from build123d import *

# Parameters (mm, degrees)
IZIM1_R                     = 10
Y_KSEKLIK_EKSTR_ZYON1_DEPTH = 25
RADYUS1_R                   = 20
RADYUS2_R                   = 100
PAH1_SIZE                   = 2
KES_EKSTR_ZYON1_DEPTH       = 276.643654753
KES_EKSTR_ZYON1_DEPTH_BACK  = 276.643654753
RADYUS3_R                   = 3


with BuildPart() as part:
    # Çizim1 → Yükseklik-Ekstrüzyon1 (new body)
    with BuildSketch(Plane.XY):
        with BuildLine():
            Line((-37.396370289, 12.396370289), (-12.396370289, 12.396370289))
            Line((-12.396370289, 12.396370289), (12.396370289, -12.396370289))
            Line((12.396370289, -12.396370289), (12.396370289, -182.396370289))
            Line((12.396370289, -182.396370289), (47.759074277, -243.646370289))
            ThreePointArc((47.759074277, -243.646370289), (41.353629711, -267.551814855), (17.448185145, -261.146370289))
            Line((17.448185145, -261.146370289), (-33.791651246, -172.396370289))
            Line((-33.791651246, -172.396370289), (-12.603629711, -154.617509234))
            Line((-12.603629711, -154.617509234), (-12.603629711, -57.396370289))
            Line((-12.603629711, -57.396370289), (-37.396370289, -32.603629711))
            Line((-37.396370289, -32.603629711), (-37.396370289, 12.396370289))
        make_face()
        with Locations((-7.396370289, -177.396370289)):
            Circle(IZIM1_R, mode=Mode.SUBTRACT)
        with Locations((32.603629711, -252.396370289)):
            Circle(IZIM1_R, mode=Mode.SUBTRACT)
    extrude(amount=Y_KSEKLIK_EKSTR_ZYON1_DEPTH)

    # Radyus1
    radyus1_edges = [part.edges().sort_by_distance(p)[0] for p in [
        (-33.791651246, -172.396370289, 12.5),
        (-12.603629711, -154.617509234, 12.5),
        (-12.603629711, -57.396370289, 12.5),
    ]]
    fillet(radyus1_edges, radius=RADYUS1_R)

    # Radyus2
    radyus2_edges = [part.edges().sort_by_distance(p)[0] for p in [
        (12.396370289, -182.396370289, 12.5),
    ]]
    fillet(radyus2_edges, radius=RADYUS2_R)

    # Pah1
    pah1_edges = [part.edges().sort_by_distance(p)[0] for p in [
        (-17.396370289, -177.396370289, 0),
        (-17.396370289, -177.396370289, 25),
        (22.603629711, -252.396370289, 0),
        (22.603629711, -252.396370289, 25),
    ]]
    chamfer(pah1_edges, length=PAH1_SIZE)

    # Çizim2 → Kes-Ekstrüzyon1 (cut, two sides: drawn at the far end of the back side and taken through both)
    with BuildSketch(Plane(origin=(0, 0, 0), x_dir=(-1, 0, 0), z_dir=(0, 0, -1)).offset(-KES_EKSTR_ZYON1_DEPTH_BACK)):
        Polygon((37.396370289, 12.396370289), (37.396370289, 10.396370289), (35.896370289, 8.896370289), (37.396370289, 7.396370289), (37.396370289, 5.396370289), (35.896370289, 3.896370289), (37.396370289, 2.396370289), (37.396370289, 0.396370289), (35.896370289, -1.103629711), (37.396370289, -2.603629711), (37.396370289, -4.603629711), (35.896370289, -6.103629711), (37.396370289, -7.603629711), (37.396370289, -9.603629711), (35.896370289, -11.103629711), (37.396370289, -12.603629711), (37.396370289, -14.603629711), (35.896370289, -16.103629711), (37.396370289, -17.603629711), (37.396370289, -19.603629711), (35.896370289, -21.103629711), (37.396370289, -22.603629711), (37.396370289, -24.603629711), (35.896370289, -26.103629711), (37.396370289, -27.603629711), (37.396370289, -29.603629711), (35.896370289, -31.103629711), (37.396370289, -32.603629711), (40.97255524, -32.603629711), (40.97255524, 12.396370289), align=None)
    extrude(amount=KES_EKSTR_ZYON1_DEPTH + KES_EKSTR_ZYON1_DEPTH_BACK, mode=Mode.SUBTRACT)

    # Radyus3
    radyus3_edges = [part.edges().sort_by_distance(p)[0] for p in [
        (-27.928932188, -42.071067812, 25),
        (-14.126039061, -58.026972889, 25),
        (-12.603629711, -105.485998804, 25),
        (-14.47747397, -153.743721305, 25),
        (-20.341888285, -161.110679149, 25),
        (-27.776301919, -173.457038674, 25),
        (-3.976234895, -224.038186258, 25),
        (41.353629711, -267.551814855, 25),
        (36.776452094, -224.623910668, 25),
        (15.80378766, -181.483355556, 25),
        (-27.928932188, -42.071067812, 0),
        (-14.126039061, -58.026972889, 0),
        (-12.603629711, -105.485998804, 0),
        (-14.47747397, -153.743721305, 0),
        (-20.341888285, -161.110679149, 0),
        (-27.776301919, -173.457038674, 0),
        (-3.976234895, -224.038186258, 0),
        (41.353629711, -267.551814855, 0),
        (36.776452094, -224.623910668, 0),
        (15.80378766, -181.483355556, 0),
        (12.396370289, -83.998910668, 25),
        (0, 0, 25),
        (-24.896370289, 12.396370289, 25),
        (-24.896370289, 12.396370289, 0),
        (12.396370289, -83.998910668, 0),
        (0, 0, 0),
    ]]
    fillet(radyus3_edges, radius=RADYUS3_R)


solid = part.part
Verification items for the finished model (mm, model axes). A direction names the side the tool comes from. Coordinates: 2 decimals unless noted, no trailing zeros. Loops run counter-clockwise (first coordinate to the right, second up) from the corner with the lowest first, then second, coordinate; pieces in that order, holes last. Notation, with made-up numbers: M 75.5,-21 L 92.5,-21 A27 ccw 92.5,-1 Z; hole C 50,63.5 d9. An arc over 180 degrees is marked long. One line per item, written item: value.
1. Gauge pin test, flat ends, axial feed: P1, Ø3, axis at x = -19, y = -179.5, coming from the +Z side; P2, Ø10, axis at x = 19.5, z = 5.5, coming from the -Y side; P3, Ø9.5, axis at y = -117, z = 8, coming from the -X side; P4, Ø1, axis at x = 37.5, z = 20, coming from the +Y side. Record the tip position at first contact, or that the pin passes through.
Answers follow:
P1: z = 25
P2: y = -267.91
P3: x = -12.6
P4: y = -225.01
2. Mould release check, pull along Y, two halves, no side actions. Record for faces 3 (the cylindrical face through (-14.168, -57.926, 12.633)), 4 (the cylindrical face through (-28.5, -40.23, 0.86)), 5 (the flat face through (-25, 12.396, 12)), 6 (the flat face through (12.396, -83, 12)): pulls with the +Y half, pulls with the -Y half, needs draft (parallel to the pull), parting line crosses it, or undercut.
Answers follow:
face 3: undercut
face 4: undercut
face 5: pulls with the +Y half
face 6: needs draft
3. Section check B-B on z = 7.75. Give the number of separate pieces and of enclosed holes in the cut face, plus the area to 3 significant figures.
Answers follow:
separate pieces: 1
enclosed holes: 2
area: 9,040 mm^2
4. Section check A-A on y = -92. Record the cut outline in (x, z).
Answers follow:
outline: M -12.6,3 A3 ccw -9.6,0 L 9.4,0 A3 ccw 12.4,3 L 12.4,22 A3 ccw 9.4,25 L -9.6,25 A3 ccw -12.6,22 Z
5. Set-up check for faces 1 (the conical face through (-1.953, -168.859, 23.125)), 2 (the cylindrical face through (-28.53, -40.26, 24.1)): record each of +Z, -Z, +X, -X, +Y, -Y from which the full face is reachable in a straight line by a thin tool's end or side.
Answers follow:
face 1: +Z
face 2: +Z, -X
6. Material ranges on line 1 along Y through (x, z) = (-9, 7.5); line 2 along Y through (x, z) = (41.5, 2.75); line 3 along Y through (x, z) = (-15, 23.5), recorded low to high. Write a range as from..to.
Answers follow:
line 1: -215.34..-187.27, -167.53..9
line 2: -267.45..-256.96, -247.83..-232.83
line 3: -204.14..-184.64, -170.16..-155.6, -55.37..11.99
